Input: part model. Units: mm. Frame: model coordinates. A direction names the side the tool comes from. Coordinates: 2 decimals unless noted, no trailing zeros. Write each loop counter-clockwise with the first axis right and the second up, starting at its lowest first coordinate (ties: lowest second). Pieces come first, ordered by that corner, then holes. Notation, with made-up numbers: (25.25, -8.5) - (58.25, -8.5) arc R17 cw to (58.25, 6.5) - close; hole circle Ø5 at (17.25, 56.25). An arc over 180 degrees is marked (long way). Use CSV: the item, a comma, the result in double quotes.
```python
from build123d import *

# Parameters (mm, degrees)
SKETCH_1_R      = 3
SKETCH_1_R_2    = 6
EXTRUDE_1_DEPTH = 3
FILLET_1_R      = 5


with BuildPart() as part:
    # Sketch 1 → Extrude 1 (new body)
    with BuildSketch(Plane.XY):
        with BuildLine():
            Line((0, 0), (0, -46))
            Line((0, -46), (18, -46))
            Line((18, -46), (18, 0))
            ThreePointArc((18, 0), (26.133778881, 69.862314787), (55, 134))
            ThreePointArc((55, 134), (-3.509871984, 79.727932531), (0, 0))
        make_face()
        with Locations((9, -40)):
            Circle(SKETCH_1_R, mode=Mode.SUBTRACT)
        with Locations((9, 0)):
            Circle(SKETCH_1_R_2, mode=Mode.SUBTRACT)
    extrude(amount=EXTRUDE_1_DEPTH)

    # Fillet 1
    fillet_1_edges = [part.edges().sort_by_distance(p)[0] for p in [
        (18, -46, 1.5),
        (0, -46, 1.5),
    ]]
    fillet(fillet_1_edges, radius=FILLET_1_R)

    # Sweep 5: sweep along a path in Sketch 14
    with BuildLine(Plane.XY.offset(1.5)) as sweep_5_path:
        ThreePointArc((55, 134), (-1.251298398, 84.80293124), (-4.517936931, 10.144447336))
    # Sketch 13 → Sweep 5 (sweep, cut)
    with BuildSketch(Plane(origin=(89.145258508, 28.985369875, 0), x_dir=(0, 0, 1), z_dir=(-0.95099279, -0.309213055, 0))):
        Polygon((1.5, 110.426315789), (-0.806867017, 103.109868349), (-0.806867017, 111.673722013), (3.806867017, 111.673722013), (3.806867017, 103.109868349), align=None)
    sweep(path=sweep_5_path.line, mode=Mode.SUBTRACT)

    # Sweep 6: sweep along a path in Sketch 16
    with BuildLine(Plane.XY.offset(1.5)) as sweep_6_path:
        Line((-0.066361056, 11.822616816), (0, 0))
    # Sketch 15 → Sweep 6 (sweep, cut)
    with BuildSketch(Plane(origin=(-3.910599214, 10.373403475, 0), x_dir=(0.935717655, 0.35274987, 0), z_dir=(-0.35274987, 0.935717655, 0))):
        Polygon((-2.121804917, 0.787609901), (-2.121804917, -3), (-2.121804917, -3.6210581), (6.078075974, -3.6210581), (-0.649060873, -1.5), (6.606310798, 0.787609901), align=None)
    sweep(path=sweep_6_path.line, mode=Mode.SUBTRACT)


solid = part.part
```
(1) Cut plane B-B on y = -18. Return loops of the section in (x, z), and give its area (3 significant figures).
Check values:
outline,"(0, 0) - (18, 0) - (18, 3) - (0, 3) - close"
area,"54.0 mm^2"
(2) Reachability of faces 4 (the flat face through (18, -21, 1)), 5 (the conical face through (3.28, 83.76, 2.93)) from +Z, -Z, +X, -X, +Y, -Y: full face, straight path, thin tool, end or side. Return the list, or none.
Check values:
face 4,"+Z, -Z, +X, -Y"
face 5,"+Z, -X"
(3) Cut plane C-C on x = 9. State how many separate pieces and enclosed holes the cut face has, and give its area (3 significant figures).
Check values:
separate pieces,"3"
enclosed holes,"0"
area,"376 mm^2"
(4) Ray query, probe 1 along X at (y, z) = (-17.5, 2.4); probe 2 along Z at (x, y) = (-7.5, 24). Return the intervals inside material, ascending. Write a range as from..to.
Check values:
probe 1,"0..18"
probe 2,"1.17..1.83"
(5) Draft query along X for faces 1 (the flat face through (0, -20, 1)), 2 (the flat face through (16, 42, 0)), 3 (the cylindrical face through (3, 0, 1)). Return one class per face: pulls with the +X half, pulls with the -X half, needs draft (parallel to the pull), parting line crosses it, or undercut.
Check values:
face 1,"pulls with the -X half"
face 2,"needs draft"
face 3,"undercut"
(6) Pin query (flat end, axial travel): pin 1 Ø1.5 at (y, z) = (-23.5, 1) entering from -X. Return the tip coordinate at first contact, or that it passes through.
Check values:
pin 1,"x = 0"
(7) Cut plane A-A on z = 2.2. Return loops of the section in (x, y).
Check values:
outline,"(-2.44, 10.93) - (-2.41, 5.01) arc R95 ccw to (0, 0) - (0, -41) arc R5 ccw to (5, -46) - (13, -46) arc R5 ccw to (18, -41) - (18, 0) arc R230 cw to (53.08, 131) arc R92.78 ccw to start; hole circle Ø12 at (9, 0); hole circle Ø6 at (9, -40)"
